Input: part model. Units: mm. Frame: model coordinates. A direction names the side the tool comes from. Give positions to 0.01 mm unless a question says otherwise; leave off trailing zeros. Write each loop counter-clockwise with the first axis right and the second up, starting at its lowest first coordinate (ties: lowest second). Pieces come first, ordered by that corner, then holes. Notation, with made-up numbers: (-34.5, 9) -> (3.5, 9) arc R12 cw to (3.5, 17) -> close; hole circle Ø3 at (16, 27.5). An arc over 180 degrees is marked (long way). Return JSON: item names as keys, results as strings. Group by question number.
Item 1: Section B-B, the plane y = 0. Return loops of the section in (x, z), then the cut area to 3 significant figures.
Item 2: Section D-D, the plane x = 8.5. Return loops of the section in (y, z), then the cut area to 3 significant figures.
Item 3: Line query: line 1 (Y direction, x = 0, z = 31); line 2 (Z direction, x = -7, y = 1.5); line 3 (Z direction, x = 2, y = -12). Output: solid intervals per line, ascending. Write a range as [from, to].
Item 4: Set-up query: faces 5 (the face through (-13, 0, 30)), 6 (the face through (5, 13, 0)), 7 (the face through (0, 0, 54.5)). Return all of +Z, -Z, +X, -X, +Y, -Y with unobstructed straight access to the full face (end or side cutting, diameter ignored); none if empty.
Item 5: Mould query, pull axis Y, two halves, no side actions, for faces 1 (the face through (-0.325, 11.536, 32.535)), 2 (the face through (-3.47, -15.62, 17.26)), 3 (the face through (0, -13, 30)), 4 (the face through (0, 2.5, 48)). Classes: released by +Y, released by -Y, zero draft, split by the parting line, or undercut.
Item 6: Pin query (flat end, axial travel): P1, Ø3.5, axis at x = 13, y = -0.5, coming from the +Z side; P2, Ø1.7, axis at x = 0.5, z = 51, coming from the +Y side; P3, Ø2.5, axis at x = 0, y = 13, coming from the +Z side; P4, Ø9.5, axis at x = 0.5, y = -4.5, coming from the +Z side. Return the tip coordinate at first contact, or that it passes through.
Item 7: Section C-C, the plane z = 7.5. Return loops of the section in (x, y), then the cut area to 3 significant figures.
Item 8: Section A-A, the plane x = 0. Return loops of the section in (y, z).
from build123d import *

# Parameters (mm, degrees)
SKETCH_1_R          = 16
EXTRUDE_1_DEPTH     = 35
SKETCH_2_R          = 10
EXTRUDE_2_DEPTH     = 3
SKETCH_3_R          = 3
EXTRUDE_3_DEPTH     = 16.5
CUT_EXTRUDE_START   = 3
SKETCH_4_W          = 9.243576196
SKETCH_4_H          = 12
CUT_EXTRUDE_1_DEPTH = 0.5
SKETCH_5_R          = 13.75
EXTRUDE_4_DEPTH     = 38
SKETCH_6_R          = 1.5
CUT_EXTRUDE_2_DEPTH = 5


with BuildPart() as part:
    # ｽｹｯﾁ1 → ﾎﾞｽ - 押し出し1 (new body)
    with BuildSketch(Plane.XY):
        Circle(SKETCH_1_R)
    extrude(amount=EXTRUDE_1_DEPTH)

    # ｽｹｯﾁ2 → ﾎﾞｽ - 押し出し2 (add)
    with BuildSketch(Plane.XY.offset(35)):
        Circle(SKETCH_2_R)
    extrude(amount=EXTRUDE_2_DEPTH)

    # ｽｹｯﾁ3 → ﾎﾞｽ - 押し出し3 (add)
    with BuildSketch(Plane.XY.offset(38)):
        Circle(SKETCH_3_R)
    extrude(amount=EXTRUDE_3_DEPTH)

    # ｽｹｯﾁ4 → ｶｯﾄ - 押し出し1 (cut)
    with BuildSketch(Plane(origin=(0, 0, 0), x_dir=(1, 0, 0), z_dir=(0, 1, 0)).offset(CUT_EXTRUDE_START)):
        with Locations((0, -48.5)):
            Rectangle(SKETCH_4_W, SKETCH_4_H)
    extrude(amount=-CUT_EXTRUDE_1_DEPTH, mode=Mode.SUBTRACT)

    # ｽｹｯﾁ5 → ﾎﾞｽ - 押し出し4 (add)
    with BuildSketch(Plane(origin=(0, 0, 0), x_dir=(-1, 0, 0), z_dir=(0, 0, -1))):
        with Locations(Location((0, 0, 0), (0, 0, 180))):
            Circle(SKETCH_5_R)
    extrude(amount=EXTRUDE_4_DEPTH)

    # ｽｹｯﾁ6 → ｶｯﾄ - 押し出し2 (cut)
    with BuildSketch(Plane.XY.offset(35)):
        with Locations((0, 13)):
            Circle(SKETCH_6_R)
        with Locations((-13, 0)):
            Circle(SKETCH_6_R)
        with Locations(Location((13, 0, 0), (0, 0, 180))):
            Circle(SKETCH_6_R)
        with Locations(Location((0, -13, 0), (0, 0, 180))):
            Circle(SKETCH_6_R)
    extrude(amount=-CUT_EXTRUDE_2_DEPTH, mode=Mode.SUBTRACT)


solid = part.part
Answer below:
{
 "1": {"outline": "(-16, 0) -> (-13.75, 0) -> (-13.75, -38) -> (13.75, -38) -> (13.75, 0) -> (16, 0) -> (16, 35) -> (14.5, 35) -> (14.5, 30) -> (11.5, 30) -> (11.5, 35) -> (10, 35) -> (10, 38) -> (3, 38) -> (3, 54.5) -> (-3, 54.5) -> (-3, 38) -> (-10, 38) -> (-10, 35) -> (-11.5, 35) -> (-11.5, 30) -> (-14.5, 30) -> (-14.5, 35) -> (-16, 35) -> close", "area": "2,290 mm2"},
 "2": {"outline": "(-13.56, 0) -> (-10.81, 0) -> (-10.81, -38) -> (10.81, -38) -> (10.81, 0) -> (13.56, 0) -> (13.56, 35) -> (5.27, 35) -> (5.27, 38) -> (-5.27, 38) -> (-5.27, 35) -> (-13.56, 35) -> close", "area": "1,800 mm2"},
 "3": {"line 1": "y = [-16, -14.5], [-11.5, 11.5], [14.5, 16]", "line 2": "z = [-38, 38]", "line 3": "z = [-38, 35]"},
 "4": {"face 5": "+Z", "face 6": "-Z", "face 7": "+Z, +X, -X, +Y, -Y"},
 "5": {"face 1": "undercut", "face 2": "split by the parting line", "face 3": "undercut", "face 4": "released by +Y"},
 "6": {"P1": "stops at z = 35", "P2": "stops at y = 2.5", "P3": "stops at z = 30", "P4": "stops at z = 54.5"},
 "7": {"outline": "circle Ø32 at (0, 0)", "area": "804 mm2"},
 "8": {"outline": "(-16, 0) -> (-13.75, 0) -> (-13.75, -38) -> (13.75, -38) -> (13.75, 0) -> (16, 0) -> (16, 35) -> (14.5, 35) -> (14.5, 30) -> (11.5, 30) -> (11.5, 35) -> (10, 35) -> (10, 38) -> (3, 38) -> (3, 42.5) -> (2.5, 42.5) -> (2.5, 54.5) -> (-3, 54.5) -> (-3, 38) -> (-10, 38) -> (-10, 35) -> (-11.5, 35) -> (-11.5, 30) -> (-14.5, 30) -> (-14.5, 35) -> (-16, 35) -> close"}
}
